Can you work these out from the model? Positions are in its coordinate system, mm. A direction names the side the tool comes from. Round coordinates to 2 decimals unless told otherwise and drop trailing zeros. Write each loop counter-clockwise with the first axis right and the second up, starting at its lowest first coordinate (ties: lowest second). Pieces come first, ordered by that corner, then holes. Notation, with made-up numbers: M -2,71.5 L 32,71.5 A28 ccw 32,94.5 Z; hole C 14.25,82.25 d3. An arc over 180 degrees is marked long. Answer as a JSON object with one key per item and string values. Group by question number.
1) Suppose I cut it at B-B, the plane y = -34.5. Write out the boundary of the cut face in (x, z).
2) Suppose I cut it at C-C, the plane y = -18. Write out the boundary of the cut face in (x, z).
3) Please list where these lines run through material, in increasing order: L1, parallel to Y at x = 25.4, z = -47; L2, parallel to X at y = -142, z = -17; L3, parallel to Z at x = 47, y = -126. Write a range as [from, to].
4) If we mould it in two halves opening along X, with no side actions, what happens to faces 1 (the cylindrical face through (24.01, -123.94, -47.67)), 2 (the flat face through (6.35, -75, -21)), 3 (the flat face through (24, -75, -50.8)), 4 (the cylindrical face through (19.016, -22.506, -47.669))? For each: +X half, -X half, draft (parallel to the pull), parting line (faces both ways), or undercut.
5) On a 3-axis mill with a long thin cutter (end or side, diameter ignored), from which of +Z, -Z, +X, -X, +Y, -Y can I reach the whole of each face in a straight line? I mean faces 5 (the cylindrical face through (50.036, -77.267, -50.076)), 6 (the flat face through (30, -75, -44.45)). Say none if no direction works.
6) I'm going to push flat-ended pins straight in: pin 1 Ø6 at (x, y) = (33, -109.5) entering from +Z; pin 2 Ø11 at (y, z) = (-95, -25.5) entering from +X. Where does each tip first touch, or does it pass through?
7) Suppose I cut it at D-D, the plane z = -14.5. Write out the boundary of the cut face in (x, y), and give its area (3 significant figures).
8) Suppose I cut it at A-A, the plane x = 25.4. Write out the boundary of the cut face in (y, z), and give its area (3 significant figures).
from build123d import *

# Parameters (mm, degrees)
F1_DEPTH = 152.4
F2_R     = 2.54
F3_R     = 4.7752
F4_R     = 6.389688
F5_DEPTH = 25.4


with BuildPart() as f1:
    # F0 (on Front) → F1 (new body)
    with BuildSketch(Plane.XZ):
        Polygon((6.35, 0), (0, 0), (0, -50.8), (50.8, -50.8), (50.8, -44.45), (6.35, -44.45), align=None)
    extrude(amount=F1_DEPTH)

    # F2
    f2_edges = [f1.edges().sort_by_distance(p)[0] for p in [
        (6.35, -76.2, 0),
        (0, -76.2, 0),
        (50.8, -76.2, -44.45),
        (50.8, -76.2, -50.8),
    ]]
    fillet(f2_edges, radius=F2_R)

    # F3
    f3_edges = [f1.edges().sort_by_distance(p)[0] for p in [
        (6.35, -76.2, -44.45),
    ]]
    fillet(f3_edges, radius=F3_R)

    # F4 (on face) → F5 (cut)
    with BuildSketch(Plane(origin=(0, 0, -50.8), x_dir=(1, 0, 0), z_dir=(0, 0, -1))):
        with Locations((25.4, 130.175)):
            Circle(F4_R)
        with Locations((25.4, 22.225)):
            Circle(F4_R)
    extrude(amount=-F5_DEPTH, mode=Mode.SUBTRACT)


solid = f1.part
Results:
{
 "1": {"outline": "M 0,-50.8 L 48.26,-50.8 A2.54 ccw 50.8,-48.26 L 50.8,-46.99 A2.54 ccw 48.26,-44.45 L 11.13,-44.45 A4.78 cw 6.35,-39.67 L 6.35,-2.54 A2.54 ccw 3.81,0 L 2.54,0 A2.54 ccw 0,-2.54 Z"},
 "2": {"outline": "M 0,-50.8 L 20.61,-50.8 L 20.61,-44.45 L 11.13,-44.45 A4.78 cw 6.35,-39.67 L 6.35,-2.54 A2.54 ccw 3.81,0 L 2.54,0 A2.54 ccw 0,-2.54 Z; M 30.19,-50.8 L 48.26,-50.8 A2.54 ccw 50.8,-48.26 L 50.8,-46.99 A2.54 ccw 48.26,-44.45 L 30.19,-44.45 Z"},
 "3": {"L1": "[-152.4, -136.56], [-123.79, -28.61], [-15.84, 0]", "L2": "[0, 6.35]", "L3": "[-50.8, -44.45]"},
 "4": {"face 1": "undercut", "face 2": "+X half", "face 3": "draft", "face 4": "undercut"},
 "5": {"face 5": "-Z, +X, +Y, -Y", "face 6": "+Z, +X, +Y, -Y"},
 "6": {"pin 1": "z = -44.45", "pin 2": "x = 6.35"},
 "7": {"outline": "M 0,-152.4 L 6.35,-152.4 L 6.35,0 L 0,0 Z", "area": "968 mm^2"},
 "8": {"outline": "M -152.4,-50.8 L -136.56,-50.8 L -136.56,-44.45 L -152.4,-44.45 Z; M -123.79,-50.8 L -28.61,-50.8 L -28.61,-44.45 L -123.79,-44.45 Z; M -15.84,-50.8 L 0,-50.8 L 0,-44.45 L -15.84,-44.45 Z", "area": "805 mm^2"}
}
